```python
from build123d import *

# Parameters (mm, degrees)
SKETCH1_W           = 152.4
SKETCH1_H           = 304.8
BOSS_EXTRUDE1_DEPTH = 25.4
SKETCH2_R           = 6.35
CUT_EXTRUDE1_DEPTH  = 19.05
SKETCH3_R           = 4.741125957
CUT_EXTRUDE2_DEPTH  = 19.05
CUT_EXTRUDE3_START  = -19.05
SKETCH8_R           = 6.35
CUT_EXTRUDE3_DEPTH  = 19.05
SKETCH9_W           = 114.3
SKETCH9_H           = 25.4
SKETCH9_H_2         = 76.2
CUT_EXTRUDE5_DEPTH  = 27.94


with BuildPart() as part:
    # Sketch1 → Boss-Extrude1 (new body)
    with BuildSketch(Plane(origin=(0, 0, 0), x_dir=(1, 0, 0), z_dir=(0, 1, 0))):
        with Locations((76.2, 152.4)):
            Rectangle(SKETCH1_W, SKETCH1_H)
    extrude(amount=BOSS_EXTRUDE1_DEPTH)

    # Sketch2 → Cut-Extrude1 (cut)
    with BuildSketch(Plane(origin=(152.4, 0, 0), x_dir=(0, 0, -1), z_dir=(1, 0, 0))):
        with Locations((19.05, 12.7)):
            Circle(SKETCH2_R)
    extrude(amount=-CUT_EXTRUDE1_DEPTH, mode=Mode.SUBTRACT)

    # Sketch3 → Cut-Extrude2 (cut)
    with BuildSketch(Plane(origin=(152.4, 0, 0), x_dir=(0, 0, -1), z_dir=(1, 0, 0))):
        with Locations((285.75, 12.7)):
            Circle(SKETCH3_R)
    extrude(amount=-CUT_EXTRUDE2_DEPTH, mode=Mode.SUBTRACT)

    # Sketch8 → Cut-Extrude3 (cut)
    with BuildSketch(Plane.ZY.offset(CUT_EXTRUDE3_START)):
        with Locations((-285.75, 12.7)):
            Circle(SKETCH8_R)
        with Locations(Location((-19.05, 12.7, 0), (0, 0, 180))):
            Circle(SKETCH8_R)
    extrude(amount=CUT_EXTRUDE3_DEPTH, mode=Mode.SUBTRACT)

    # Sketch9 → Cut-Extrude5 (cut)
    with BuildSketch(Plane(origin=(0, 0, 0), x_dir=(1, 0, 0), z_dir=(0, 1, 0))):
        with Locations((76.2, 31.75)):
            Rectangle(SKETCH9_W, SKETCH9_H)
        with Locations((76.2, 245.100072294)):
            Rectangle(SKETCH9_W, SKETCH9_H_2)
    extrude(amount=CUT_EXTRUDE5_DEPTH, mode=Mode.SUBTRACT)


solid = part.part
```
Model file for the job. Use its own axes, mm. A direction names the side the tool comes from. Coordinates: 2 decimals unless noted, no trailing zeros. Loops run counter-clockwise (first coordinate to the right, second up) from the corner with the lowest first, then second, coordinate; pieces in that order, holes last. Notation, with made-up numbers: (11.5, 82.25) - (31.5, 82.25) arc R20 cw to (31.5, 116.25) - close; hole circle Ø2 at (34, 13.5). An arc over 180 degrees is marked (long way). Answer as a JSON object with one key per item and string values. Group by question number.
(1) Cut at C-C (z = -211). Give the cut face in (x, y), then the cut area to 3 significant figures.
(2) Two-plate mould, pull along Z, no slides. Class faces 5 (the face through (75, 25.4, -155)), 6 (the face through (9.658, 12.979, -292.094)): released by +Z, released by -Z, zero draft, split by the parting line, or undercut.
(3) Cut at B-B (x = 71.5). Give the cut face in (y, z).
(4) Tool access for faces 1 (the face through (143.01, 10.88, -290.13)), 2 (the face through (9.658, 15.132, -24.916)), 3 (the face through (0, 13, -150)), 4 (the face through (75, 13, -283.2)): list every direction of +Z, -Z, +X, -X, +Y, -Y with a clear straight run to the whole face (end or side of a thin tool).
(5) Cut at A-A (y = 12.7). Give the cut face in (x, z).
(6) Flat gauge pins, fed straight in: pin 1 (6 mm diameter, centred on y = 14, z = -286.5, fed in from +X); pin 2 (5 mm diameter, centred on y = 13, z = -16, fed in from -X); pin 3 (12 mm diameter, centred on x = 126.5, z = -260, fed in from -Y). Where does each tip first touch, or does it go through?
(7) Probe line 1 along Z through (x, y) = (60, 23.5); line 2 along Z through (x, y) = (140.25, 12.7); line 3 along Y through (x, z) = (137, -19). List the from-to ranges inside material, lowest first.
Geometry says:
{
 "1": {"outline": "(0, 0) - (19.05, 0) - (19.05, 25.4) - (0, 25.4) - close; (133.35, 0) - (152.4, 0) - (152.4, 25.4) - (133.35, 25.4) - close", "area": "968 mm^2"},
 "2": {"face 5": "zero draft", "face 6": "undercut"},
 "3": {"outline": "(0, -304.8) - (25.4, -304.8) - (25.4, -283.2) - (0, -283.2) - close; (0, -207) - (25.4, -207) - (25.4, -44.45) - (0, -44.45) - close; (0, -19.05) - (25.4, -19.05) - (25.4, 0) - (0, 0) - close"},
 "4": {"face 1": "+X", "face 2": "-X", "face 3": "+Z, -Z, -X, +Y, -Y", "face 4": "+Y, -Y"},
 "5": {"outline": "(0, -304.8) - (152.4, -304.8) - (152.4, -290.49) - (133.35, -290.49) - (133.35, -283.2) - (19.05, -283.2) - (19.05, -292.1) - (0, -292.1) - close; (0, -279.4) - (19.05, -279.4) - (19.05, -207) - (133.35, -207) - (133.35, -281.01) - (152.4, -281.01) - (152.4, -25.4) - (133.35, -25.4) - (133.35, -44.45) - (19.05, -44.45) - (19.05, -25.4) - (0, -25.4) - close; (0, -12.7) - (19.05, -12.7) - (19.05, -19.05) - (133.35, -19.05) - (133.35, -12.7) - (152.4, -12.7) - (152.4, 0) - (0, 0) - close"},
 "6": {"pin 1": "stops at x = 133.35", "pin 2": "stops at x = 19.05", "pin 3": "passes through"},
 "7": {"line 1": "z = -304.8 to -283.2, -207 to -44.45, -19.05 to 0", "line 2": "z = -304.8 to -290.49, -281.01 to -25.4, -12.7 to 0", "line 3": "y = 0 to 6.35, 19.05 to 25.4"}
}
